Design review of the part built by this model. Coordinates are the model's own, in mm. A direction names the side the tool comes from. Coordinates: 2 decimals unless noted, no trailing zeros. Order: outer loops, then holes, each group sorted by start corner. A loop starts at its lowest first (then second) coordinate and runs counter-clockwise, first axis right, second up. Notation, with made-up numbers: (53.5, 16) -> (112.5, 16) arc R16 ccw to (112.5, 27) -> close; hole circle Ø1 at (30.25, 28). An arc over 180 degrees is marked (long way). Write item = value, one per line.
```python
from build123d import *

# Parameters (mm, degrees)
SKETCH1_W            = 6.858
SKETCH1_H            = 6.858
BOSS_EXTRUDE1_DEPTH  = 6.858
CUT_EXTRUDE1_DEPTH   = 6.858
BOSS_EXTRUDE2_DEPTH  = 12.7
MOVE_FACE1_BY        = 0.889
MOVE_START           = 68.758370303
MOVE_FACE2_OUTLINE_W = 1.27
MOVE_FACE2_OUTLINE_H = 5.969
MOVE_FACE2_DEPTH     = 6.858
MOVE_FACE3_BY        = 1.27


# Read off the part's stored shape, not the designer's step: Move Face2
with BuildPart() as part:
    # Sketch1 → Boss-Extrude1 (new body)
    with BuildSketch(Plane.XY):
        with Locations((72.187370303, 7.35377716)):
            Rectangle(SKETCH1_W, SKETCH1_H)
    extrude(amount=BOSS_EXTRUDE1_DEPTH)

    # Sketch3 → Cut-Extrude1 (cut)
    with BuildSketch(Plane.XY.offset(6.858)):
        with BuildLine():
            ThreePointArc((73.987370303, 7.35377716), (72.187370303, 9.15377716), (70.387370303, 7.35377716))
            Line((70.387370303, 7.35377716), (73.987370303, 7.35377716))
        make_face()
        with BuildLine():
            Line((73.987370303, 7.35377716), (70.387370303, 7.35377716))
            ThreePointArc((70.387370303, 7.35377716), (72.187370303, 5.55377716), (73.987370303, 7.35377716))
        make_face()
    extrude(amount=-CUT_EXTRUDE1_DEPTH, mode=Mode.SUBTRACT)

    # Sketch5 → Boss-Extrude2 (add)
    with BuildSketch(Plane(origin=(0, 10.78277716, 0), x_dir=(1, 0, 0), z_dir=(0, 1, 0))):
        with BuildLine():
            ThreePointArc((72.187370303, -0.889), (69.647370303, -3.429), (72.187370303, -5.969))
            Line((72.187370303, -5.969), (72.187370303, -0.889))
        make_face()
        with BuildLine():
            Line((72.187370303, -0.889), (72.187370303, -5.969))
            ThreePointArc((72.187370303, -5.969), (73.983421527, -5.225051224), (74.727370303, -3.429))
            ThreePointArc((74.727370303, -3.429), (73.983421527, -1.632948776), (72.187370303, -0.889))
        make_face()
    extrude(amount=BOSS_EXTRUDE2_DEPTH)

    # Move Face1: a face moved inward by 0.889
    extrude(part.faces().sort_by_distance((72.187370303, 4.61057716, 6.858))[0], amount=MOVE_FACE1_BY, dir=(0, 0, -1), mode=Mode.SUBTRACT)

    # Move Face2 outline → Move Face2 (add)
    with BuildSketch(Plane.YZ.offset(MOVE_START)):
        with Locations((11.41777716, 2.9845)):
            Rectangle(MOVE_FACE2_OUTLINE_W, MOVE_FACE2_OUTLINE_H)
    extrude(amount=MOVE_FACE2_DEPTH)

    # Move Face3: a face moved outward by 1.27
    extrude(part.faces().sort_by_distance((72.187370303, 23.48277716, 3.429))[0], amount=MOVE_FACE3_BY, dir=(0, 1, 0))


solid = part.part
```
(1) We need section A-A (z = 4.5). Write out the cut boundary in (x, y), and give its area (3 significant figures).
Report:
outline = (68.76, 3.92) -> (75.62, 3.92) -> (75.62, 12.05) -> (74.49, 12.05) -> (74.49, 24.75) -> (69.88, 24.75) -> (69.88, 12.05) -> (68.76, 12.05) -> close; hole circle Ø3.6 at (72.19, 7.35)
area = 104 mm²
(2) Insertion check: pin 1 (2 mm diameter, centred on x = 75, y = 16, fed in from +Z); pin 2 (3 mm diameter, centred on x = 73, y = 17.5, fed in from -Z); pin 3 (1.5 mm diameter, centred on y = 18, z = 3.5, fed in from -X). Each pin has a flat end and moves straight along its axis. Give the tip position at first contact, or say it passes through.
Report:
pin_1 = 5.21
pin_2 = 0.89
pin_3 = 69.65
(3) The part is to be moulded in two halves that separate along X. For faces 3 (the flat face through (72, 3.925, 3)), 4 (the flat face through (68.758, 8, 3)), 5 (the cylindrical face through (70.47, 6.81, 3.03)), say which applies: released by +X, released by -X, zero draft, split by the parting line, or undercut.
Report:
face_3 = zero draft
face_4 = released by -X
face_5 = undercut
(4) For faces 1 (the cylindrical face through (72.3, 18.31, 0.89)), 2 (the flat face through (72, 24.753, 3)), list the 3-axis set-ups (+Z, -Z, +X, -X, +Y, -Y) from which the entire face can be reached by the end or side of a thin tool; tool diameter is ignored.
Report:
face_1 = +Y
face_2 = +Z, -Z, +X, -X, +Y
(5) For L1, parallel to Y at x = 69.5, z = 0.4; L2, parallel to X at y = 18.75, z = 3.35; L3, parallel to X at y = 8, z = 4.1, list the stretches that pass through material, from the lowest coordinate up.
Report:
L1 = 3.92 to 12.05
L2 = 69.65 to 74.73
L3 = 68.76 to 70.51, 73.87 to 75.62
(6) We need section C-C (y = 6.75). Write out the cut boundary in (x, z).
Report:
outline = (68.76, 0) -> (70.49, 0) -> (70.49, 5.97) -> (68.76, 5.97) -> close; (73.88, 0) -> (75.62, 0) -> (75.62, 5.97) -> (73.88, 5.97) -> close
(7) We need section D-D (z = 1.4). Write out the cut boundary in (x, y).
Report:
outline = (68.76, 3.92) -> (75.62, 3.92) -> (75.62, 12.05) -> (73.72, 12.05) -> (73.72, 24.75) -> (70.66, 24.75) -> (70.66, 12.05) -> (68.76, 12.05) -> close; hole circle Ø3.6 at (72.19, 7.35)
